Can you work these out from the model? Positions are in its coordinate system, mm. A direction names the side the tool comes from. Give positions to 0.01 mm unless a question says otherwise; leave off trailing zeros. Loops run counter-clockwise (first coordinate to the right, second up) from the corner with the lowest first, then second, coordinate; pieces in that order, holes last. Notation, with made-up numbers: M 42.5,30 L 92.5,30 A30 cw 92.5,60 Z; hole C 0,-26 d8. An arc over 180 degrees is marked long. Answer as a JSON object with one key per item and string values.
```python
from build123d import *

# Parameters (mm, degrees)
SKETCH1_R           = 7.736199
SKETCH1_R_2         = 5
SKETCH1_R_3         = 2.5
BOSS_EXTRUDE1_DEPTH = 2
BOSS_EXTRUDE4_START = 21.349633
SKETCH2_W           = 92
SKETCH2_H           = 110
BOSS_EXTRUDE4_DEPTH = 2
SKETCH4_W           = 110
SKETCH4_H           = 87
BOSS_EXTRUDE5_DEPTH = 2
BOSS_EXTRUDE6_START = -165.340784
BOSS_EXTRUDE6_DEPTH = 2
BOSS_EXTRUDE8_START = 115.349633
SKETCH7_W           = 42.046546
SKETCH7_H           = 18.25
BOSS_EXTRUDE8_DEPTH = 2


with BuildPart() as part:
    # Sketch1 → Boss-Extrude1 (new body)
    with BuildSketch(Plane.XY):
        with BuildLine():
            Line((-73.340784, 141.349633), (-73.340784, 21.349633))
            Line((-73.340784, 21.349633), (-119.340784, 21.349633))
            Line((-119.340784, 21.349633), (-165.340784, 21.349633))
            Line((-165.340784, 21.349633), (-165.340784, 31.349633))
            Line((-165.340784, 31.349633), (-165.340784, 111.349633))
            Line((-165.340784, 111.349633), (-119.340784, 111.349633))
            Line((-119.340784, 111.349633), (-119.340784, 141.349633))
            ThreePointArc((-119.340784, 141.349633), (-96.340784, 164.349633), (-73.340784, 141.349633))
        make_face()
        with Locations((-96.340784, 141.349633)):
            Circle(SKETCH1_R, mode=Mode.SUBTRACT)
        with Locations((-85.340784, 101.349633)):
            Circle(SKETCH1_R_2, mode=Mode.SUBTRACT)
        with Locations((-77.819625, 141.785505)):
            Circle(SKETCH1_R_3, mode=Mode.SUBTRACT)
        with Locations((-114.840784, 141.349633)):
            Circle(SKETCH1_R_3, mode=Mode.SUBTRACT)
        with Locations((-155.340784, 101.349633)):
            Circle(SKETCH1_R_2, mode=Mode.SUBTRACT)
        with Locations((-85.340784, 31.349633)):
            Circle(SKETCH1_R_2, mode=Mode.SUBTRACT)
        with Locations((-155.340784, 31.349633)):
            Circle(SKETCH1_R_2, mode=Mode.SUBTRACT)
    extrude(amount=BOSS_EXTRUDE1_DEPTH)



with BuildPart() as body_2:
    # Sketch2 → Boss-Extrude4 (new body)
    with BuildSketch(Plane(origin=(0, 0, 0), x_dir=(1, 0, 0), z_dir=(0, 1, 0)).offset(BOSS_EXTRUDE4_START)):
        with Locations((-119.340784, -55)):
            Rectangle(SKETCH2_W, SKETCH2_H)
    extrude(amount=-BOSS_EXTRUDE4_DEPTH)


with BuildPart() as part_1:
    add(part.part)

    add(body_2.part)  # Boss-Extrude5 merges body 2
    # Sketch4 → Boss-Extrude5 (add)
    with BuildSketch(Plane(origin=(-73.340784, 0, 0), x_dir=(0, 0, -1), z_dir=(1, 0, 0))):
        with Locations((-55, 62.849633)):
            Rectangle(SKETCH4_W, SKETCH4_H)
    extrude(amount=-BOSS_EXTRUDE5_DEPTH)

    # Sketch5 → Boss-Extrude6 (add)
    with BuildSketch(Plane(origin=(0, 0, 0), x_dir=(0, 0, -1), z_dir=(1, 0, 0)).offset(BOSS_EXTRUDE6_START)):
        Polygon((0, 19.349633), (-110, 19.349633), (-110, 106.349633), (-32, 106.349633), (-32, 115.349633), (-13.75, 115.349633), (-13.75, 111.349633), (0, 111.349633), (0, 106.349633), align=None)
    extrude(amount=-BOSS_EXTRUDE6_DEPTH)

    # Sketch7 → Boss-Extrude8 (add)
    with BuildSketch(Plane(origin=(0, 0, 0), x_dir=(1, 0, 0), z_dir=(0, 1, 0)).offset(BOSS_EXTRUDE8_START)):
        with Locations((-186.364057, -22.875)):
            Rectangle(SKETCH7_W, SKETCH7_H)
    extrude(amount=-BOSS_EXTRUDE8_DEPTH)


solid = part_1.part
```
1) Suppose I cut it at C-C, the plane y = 90.5. Write out the boundary of the cut face in (x, z), and give its area (3 significant figures).
Answer list:
{"outline": "M -167.34,0 L -73.34,0 L -73.34,110 L -75.34,110 L -75.34,2 L -165.34,2 L -165.34,110 L -167.34,110 Z", "area": "620 mm^2"}
2) Will these pins go through, and if not, where does the flat tip stop? pin 1 Ø20 at (x, z) = (-181.5, 27) entering from -Y; pin 2 Ø20 at (x, z) = (-180, 21) entering from +Y; pin 3 Ø16 at (x, y) = (-155.34, 31.35) entering from +Z; pin 4 Ø6 at (x, y) = (-85.34, 101.35) entering from -Z.
Answer list:
{"pin 1": "y = 113.35", "pin 2": "y = 115.35", "pin 3": "z = 2", "pin 4": "through"}
3) Suppose I cut it at B-B, the plane x = -86.5. Write out the boundary of the cut face in (y, z), and give its area (3 significant figures).
Answer list:
{"outline": "M 19.35,0 L 26.49,0 L 26.49,2 L 21.35,2 L 21.35,110 L 19.35,110 Z; M 36.21,0 L 96.49,0 L 96.49,2 L 36.21,2 Z; M 106.21,0 L 162.14,0 L 162.14,2 L 106.21,2 Z", "area": "463 mm^2"}
4) Please list where these lines run through material, in increasing order: line 1 along X through (y, z) = (65, 102.5); line 2 along Y through (x, z) = (-105, 85); line 3 along Z through (x, y) = (-101, 25.5). Write a range as from..to.
Answer list:
{"line 1": "-167.34..-165.34, -75.34..-73.34", "line 2": "19.35..21.35", "line 3": "0..2"}
5) Suppose I cut it at D-D, the plane x = -136. Write out the boundary of the cut face in (y, z).
Answer list:
{"outline": "M 19.35,0 L 111.35,0 L 111.35,2 L 21.35,2 L 21.35,110 L 19.35,110 Z"}
6) If we mould it in two halves opening along X, with no side actions, what happens to faces 1 (the flat face through (-73.341, 68, 56)), 2 (the cylindrical face through (-156.425, 96.469, 0.986)), 3 (the flat face through (-187, 114, 13.75)), 4 (the cylindrical face through (-79.66, 143.48, 0.99))? For each: +X half, -X half, draft (parallel to the pull), parting line (faces both ways), or undercut.
Answer list:
{"face 1": "+X half", "face 2": "undercut", "face 3": "draft", "face 4": "undercut"}
7) Suppose I cut it at A-A, the plane z = 60. Write out the boundary of the cut face in (x, y), and give its area (3 significant figures).
Answer list:
{"outline": "M -167.34,19.35 L -73.34,19.35 L -73.34,106.35 L -75.34,106.35 L -75.34,21.35 L -165.34,21.35 L -165.34,106.35 L -167.34,106.35 Z", "area": "528 mm^2"}
8) For faces 5 (the cylindrical face through (-96.847, 164.344, 0.986)), 6 (the flat face through (-185, 114, 32)), 7 (the flat face through (-147, 111.35, 1)), 8 (the flat face through (-75.341, 64, 57)), 9 (the flat face through (-188, 113.35, 23)), which set-ups out of +Z, -Z, +X, -X, +Y, -Y let a thin tool reach every point of the face, with its end or its side?
Answer list:
{"face 5": "+Z, -Z, +Y", "face 6": "+Z, +X, -X, +Y", "face 7": "-Z, -X, +Y", "face 8": "+Z, +Y", "face 9": "+Z, -Z, -X, -Y"}
